Study the drawing (mm; zero at the part's minimum x, y, z) and answer. A direction names the side the tool comes from. Coordinates: 2 decimals unless noted, no trailing zeros. Loops run counter-clockwise (first coordinate to the right, second up) from the corner with the lowest first, then second, coordinate; pieces in that order, holes last. Notation, with made-up numbers: (0, 89.25) -> (17, 89.25) arc R19 ccw to (17, 126.25) -> close; hole circle Ø3 at (52.25, 68.5). An arc over 180 degrees is marked (long way). Answer as a JSON object with one key per item and string values. Group by question number.
Q1. The part is cut by section A-A on y = 0.7. Write down the section's boundary in (x, z) (1 decimal).
Q2. Determine the mould class of the marked faces 1 and 2 for opening direction X: released by +X, released by -X, zero draft, split by the parting line, or undercut.
Q3. The part is cut by section D-D on z = 0.55. Write down the section's boundary in (x, y).
Q4. The part is cut by section B-B on x = 2.25. Write down the section's boundary in (y, z) (1 decimal).
Q5. Each of these flat-tipped pins is pushed along its axis until it touches: P1, Ø1.5, axis at y = 0.5, z = 1.5, coming from the +X side; P2, Ø1.5, axis at x = 13.5, y = 0.5, coming from the -Z side. Where does it stop, or does it pass through?
Q6. The part is cut by section C-C on z = 1.9. Write down the section's boundary in (x, y) (1 decimal).
Q7. Straight lines are drawn through the part: line 1 along X through (y, z) = (2.1, 1.5); line 2 along X through (y, z) = (1.45, 1.45) (1 decimal); line 3 along Z through (x, y) = (8.5, 2.25) (1 decimal). For each, find the intervals that lie inside material, in ascending order. Write a range as [from, to].
Q8. For the marked faces 3, 4 and 5, determine the directions among +Z, -Z, +X, -X, +Y, -Y from which every point of the face is accessible in a straight line to the end or side of a thin tool.
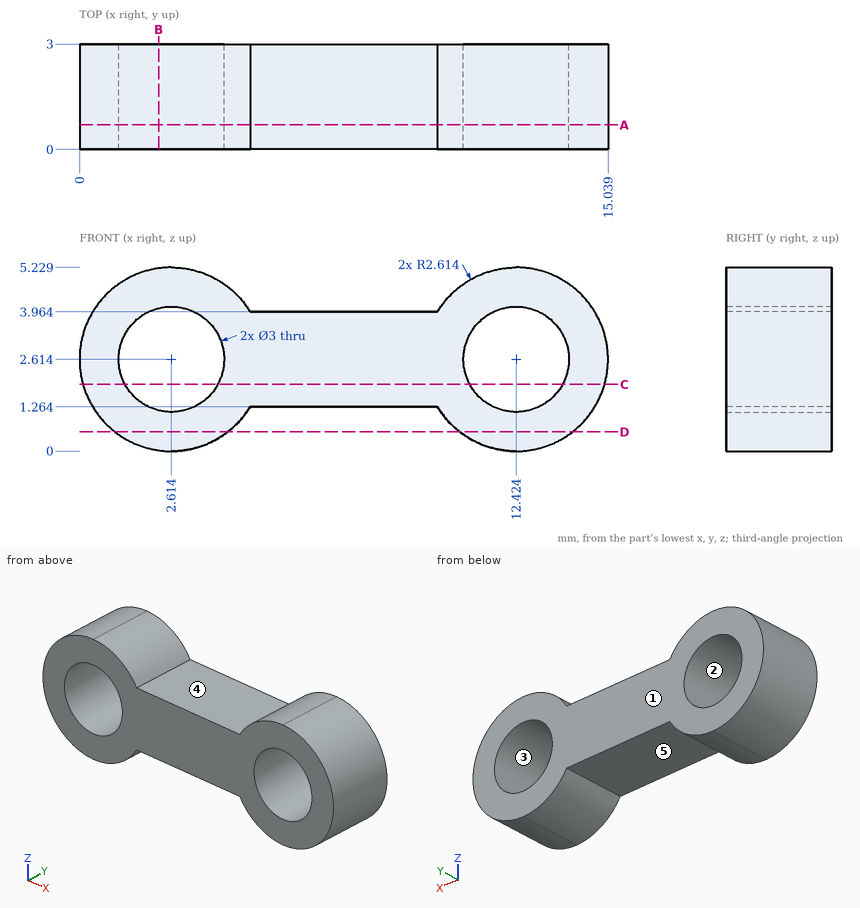
Final values:
{
 "1": {"outline": "(4.9, 1.3) -> (10.2, 1.3) arc R2.6 ccw (long way) to (10.2, 4) -> (4.9, 4) arc R2.6 ccw (long way) to start; hole circle Ø3 at (2.6, 2.6); hole circle Ø3 at (12.4, 2.6)"},
 "2": {"face 1": "zero draft", "face 2": "undercut"},
 "3": {"outline": "(1.01, 0) -> (4.22, 0) -> (4.22, 3) -> (1.01, 3) -> close; (10.82, 0) -> (14.03, 0) -> (14.03, 3) -> (10.82, 3) -> close"},
 "4": {"outline": "(0, 0) -> (3, 0) -> (3, 1.2) -> (0, 1.2) -> close; (0, 4.1) -> (3, 4.1) -> (3, 5.2) -> (0, 5.2) -> close"},
 "5": {"P1": "stops at x = 15.01", "P2": "stops at z = 0.02"},
 "6": {"outline": "(0.1, 0) -> (1.3, 0) -> (1.3, 3) -> (0.1, 3) -> close; (3.9, 0) -> (11.1, 0) -> (11.1, 3) -> (3.9, 3) -> close; (13.7, 0) -> (14.9, 0) -> (14.9, 3) -> (13.7, 3) -> close"},
 "7": {"line 1": "x = [0.25, 1.61], [3.62, 11.42], [13.43, 14.79]", "line 2": "x = [0.3, 1.7], [3.6, 11.5], [13.4, 14.8]", "line 3": "z = [1.3, 4]"},
 "8": {"face 3": "+Y, -Y", "face 4": "+Z, +Y, -Y", "face 5": "-Z, +Y, -Y"}
}
